```python
from build123d import *

# Parameters (mm, degrees)
SKETCH1_R           = 3.25
BOSS_EXTRUDE1_DEPTH = 10
CUT_EXTRUDE1_DEPTH  = 7
SKETCH3_R           = 2.5
CUT_EXTRUDE2_DEPTH  = 10
FILLET1_R           = 3.5


with BuildPart() as part:
    # Sketch1 → Boss-Extrude1 (new body)
    with BuildSketch(Plane.XY):
        with BuildLine():
            Line((-73.747603834, 33.92172524), (58.252396166, 33.92172524))
            ThreePointArc((58.252396166, 33.92172524), (61.080823291, 32.750152364), (62.252396166, 29.92172524))
            Line((62.252396166, 29.92172524), (62.252396166, -17.07827476))
            ThreePointArc((62.252396166, -17.07827476), (61.080823291, -19.906701885), (58.252396166, -21.07827476))
            Line((58.252396166, -21.07827476), (-73.747603834, -21.07827476))
            ThreePointArc((-73.747603834, -21.07827476), (-76.576030959, -19.906701885), (-77.747603834, -17.07827476))
            Line((-77.747603834, -17.07827476), (-77.747603834, 29.92172524))
            ThreePointArc((-77.747603834, 29.92172524), (-76.576030959, 32.750152364), (-73.747603834, 33.92172524))
        make_face()
        with Locations((-22.747603834, 10.92172524)):
            Circle(SKETCH1_R, mode=Mode.SUBTRACT)
    extrude(amount=BOSS_EXTRUDE1_DEPTH)

    # Sketch2 → Cut-Extrude1 (cut)
    with BuildSketch(Plane.XY.offset(10)):
        with BuildLine():
            Line((-77.747603834, 23.92172524), (-71.247603834, 23.92172524))
            ThreePointArc((-71.247603834, 23.92172524), (-68.7727301, 24.946851505), (-67.747603834, 27.42172524))
            Line((-67.747603834, 27.42172524), (-67.747603834, 33.92172524))
            Line((-67.747603834, 33.92172524), (-77.747603834, 33.92172524))
            Line((-77.747603834, 33.92172524), (-77.747603834, 23.92172524))
        make_face()
        with BuildLine():
            Line((-77.747603834, -11.07827476), (-71.247603834, -11.07827476))
            ThreePointArc((-71.247603834, -11.07827476), (-68.7727301, -12.103401026), (-67.747603834, -14.57827476))
            Line((-67.747603834, -14.57827476), (-67.747603834, -21.07827476))
            Line((-67.747603834, -21.07827476), (-77.747603834, -21.07827476))
            Line((-77.747603834, -21.07827476), (-77.747603834, -11.07827476))
        make_face()
        with BuildLine():
            Line((52.252396166, -21.07827476), (62.252396166, -21.07827476))
            Line((62.252396166, -21.07827476), (62.252396166, -11.07827476))
            Line((62.252396166, -11.07827476), (55.752396166, -11.07827476))
            ThreePointArc((55.752396166, -11.07827476), (53.277522432, -12.103401026), (52.252396166, -14.57827476))
            Line((52.252396166, -14.57827476), (52.252396166, -21.07827476))
        make_face()
        with BuildLine():
            Line((62.252396166, 23.92172524), (55.752396166, 23.92172524))
            ThreePointArc((55.752396166, 23.92172524), (53.277522432, 24.946851505), (52.252396166, 27.42172524))
            Line((52.252396166, 27.42172524), (52.252396166, 33.92172524))
            Line((52.252396166, 33.92172524), (62.252396166, 33.92172524))
            Line((62.252396166, 33.92172524), (62.252396166, 23.92172524))
        make_face()
    extrude(amount=-CUT_EXTRUDE1_DEPTH, mode=Mode.SUBTRACT)

    # Sketch3 → Cut-Extrude2 (cut)
    with BuildSketch(Plane.XY.offset(3)):
        with Locations((-72.747603834, 28.92172524)):
            Circle(SKETCH3_R)
        with Locations((57.252396166, 28.92172524)):
            Circle(SKETCH3_R)
        with Locations((57.252396166, -16.07827476)):
            Circle(SKETCH3_R)
        with Locations((-72.747603834, -16.07827476)):
            Circle(SKETCH3_R)
    extrude(amount=-CUT_EXTRUDE2_DEPTH, mode=Mode.SUBTRACT)

    # Fillet1
    fillet1_edges = [part.edges().sort_by_distance(p)[0] for p in [
        (52.252396166, 33.92172524, 6.5),
        (62.252396166, 23.92172524, 6.5),
        (62.252396166, -11.07827476, 6.5),
        (52.252396166, -21.07827476, 6.5),
        (-67.747603834, -21.07827476, 6.5),
        (-77.747603834, -11.07827476, 6.5),
        (-77.747603834, 23.92172524, 6.5),
        (-67.747603834, 33.92172524, 6.5),
    ]]
    fillet(fillet1_edges, radius=FILLET1_R)


solid = part.part
```
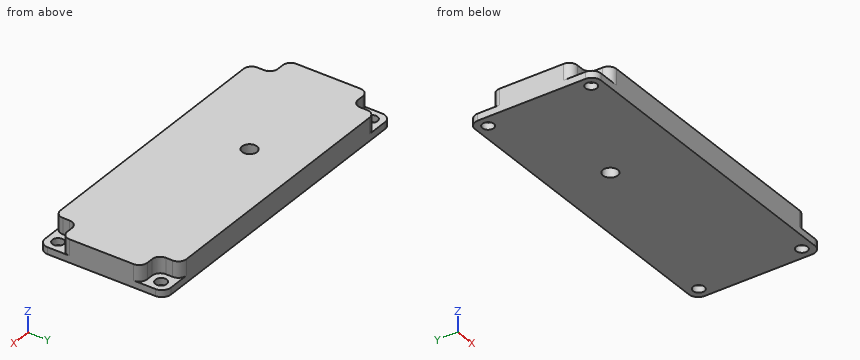
Input: part model. Units: mm. Frame: model coordinates. Round coordinates to 2 decimals unless told otherwise and drop trailing zeros. Loops run counter-clockwise (first coordinate to the right, second up) from the corner with the lowest first, then second, coordinate; pieces in that order, holes last.
1) Material intervals for line 1 (X direction, y = 29.5, z = 1.75); line 2 (X direction, y = -17.5, z = 9.5); line 3 (X direction, y = 13, z = 9), sorted ascending.
Ans:
line 1: x = -77.75 to -75.18, -70.32 to 54.82, 59.68 to 62.25
line 2: x = -67.75 to 52.25
line 3: x = -77.75 to -25.25, -20.25 to 62.25
2) Pin query (flat end, axial travel): pin 1 (1.5 mm diameter, centred on x = 56.5, z = 5, fed in from +Y); pin 2 (8 mm diameter, centred on x = -72.75, y = 28.92, fed in from +Z); pin 3 (1.5 mm diameter, centred on x = -72.5, z = 6, fed in from -Y). Return the tip coordinate at first contact, or that it passes through.
Ans:
pin 1: stops at y = 23.92
pin 2: stops at z = 3
pin 3: stops at y = -11.08
3) Section query B-B on x = -66.5. Return the cut outline in (y, z).
Ans:
outline: (-21.08, 0) - (33.92, 0) - (33.92, 3) - (33.1, 3) - (33.1, 10) - (-20.26, 10) - (-20.26, 3) - (-21.08, 3) - close
4) Section query A-A on z = 6.5. Return the cut outline in (x, y).
Ans:
outline: (-77.75, -7.58) arc R3.5 ccw to (-74.25, -11.08) - (-71.25, -11.08) arc R3.5 cw to (-67.75, -14.58) - (-67.75, -17.58) arc R3.5 ccw to (-64.25, -21.08) - (48.75, -21.08) arc R3.5 ccw to (52.25, -17.58) - (52.25, -14.58) arc R3.5 cw to (55.75, -11.08) - (58.75, -11.08) arc R3.5 ccw to (62.25, -7.58) - (62.25, 20.42) arc R3.5 ccw to (58.75, 23.92) - (55.75, 23.92) arc R3.5 cw to (52.25, 27.42) - (52.25, 30.42) arc R3.5 ccw to (48.75, 33.92) - (-64.25, 33.92) arc R3.5 ccw to (-67.75, 30.42) - (-67.75, 27.42) arc R3.5 cw to (-71.25, 23.92) - (-74.25, 23.92) arc R3.5 ccw to (-77.75, 20.42) - close; hole circle Ø6.5 at (-22.75, 10.92)
